```python
from build123d import *

# Parameters (mm, degrees)
F0_W     = 100
F0_H     = 100
F2_DEPTH = 15
F1_R     = 25
F3_DEPTH = 15.001
F4_R     = 8
F5_DEPTH = 15.001
F7_D     = 3.3
F7_DEPTH = 13.5
F7_TIP   = 0.9914200214


with BuildPart() as f2:
    # F0 (on Front) → F2 (new body)
    with BuildSketch(Plane.XZ):
        Rectangle(F0_W, F0_H)
    extrude(amount=F2_DEPTH)

    # F1 (on Front) → F3 (cut, through all)
    with BuildSketch(Plane.XZ):
        Circle(F1_R)
    extrude(amount=F3_DEPTH, mode=Mode.SUBTRACT)

    # F4 (on Front) → F5 (cut, through all)
    with BuildSketch(Plane.XZ):
        with Locations((0, 39.0632459029)):
            Circle(F4_R)
    extrude(amount=F5_DEPTH, mode=Mode.SUBTRACT)

    # F7
    with Locations(Plane.XY.offset(50)):
        with Locations((0, -8.1104654819)):
            Hole(F7_D / 2, depth=F7_DEPTH)
            with Locations((0, 0, -(F7_DEPTH + F7_TIP / 2))):  # 118° drill point
                Cone(0, F7_D / 2, F7_TIP, mode=Mode.SUBTRACT)


solid = f2.part
```
Design review of the part built by this model. Coordinates are the model's own, in mm. Coordinates: 2 decimals unless noted, no trailing zeros. Loops run counter-clockwise (first coordinate to the right, second up) from the corner with the lowest first, then second, coordinate; pieces in that order, holes last. Notation, with made-up numbers: (24.5, 79) -> (38.5, 79) arc R27 cw to (38.5, 96) -> close; hole circle Ø11 at (34.5, 83). An arc over 180 degrees is marked (long way). Answer as a JSON object with one key per item and string values.
Q1. Take a section at C-C on x = -4. Give the boundary of the cut face in (y, z).
Answer block:
{"outline": "(-15, -50) -> (0, -50) -> (0, -24.68) -> (-15, -24.68) -> close; (-15, 24.68) -> (0, 24.68) -> (0, 32.14) -> (-15, 32.14) -> close; (-15, 45.99) -> (0, 45.99) -> (0, 50) -> (-15, 50) -> close"}
Q2. The part is to be moulded in two halves that separate along X. For faces 1 (the flat face through (-50, -7, -1)), 2 (the cylindrical face through (23.846, -7.395, 7.509)), 3 (the cylindrical face through (-1.524, -8.742, 48.421)), 4 (the flat face through (-1, -6, 50)), say which applies: +X half, -X half, draft (parallel to the pull), parting line (faces both ways), or undercut.
Answer block:
{"face 1": "-X half", "face 2": "undercut", "face 3": "undercut", "face 4": "draft"}
Q3. To check wall thickness, follow L1, parallel to Y at x = 0, z = 48.05; L2, parallel to Z at x = 0, y = -12; L3, parallel to Z at x = -5, y = -2. State the ranges of each line that lie inside material, in increasing order.
Answer block:
{"L1": "y = -15 to -9.76, -6.46 to 0", "L2": "z = -50 to -25, 25 to 31.06, 47.06 to 50", "L3": "z = -50 to -24.49, 24.49 to 32.82, 45.31 to 50"}
Q4. Take a section at D-D on y = -3.75. Give the boundary of the cut face in (x, z).
Answer block:
{"outline": "(-50, -50) -> (50, -50) -> (50, 50) -> (-50, 50) -> close; hole circle Ø50 at (0, 0); hole circle Ø16 at (0, 39.06)"}
Q5. Take a section at B-B on z = 0. Give the boundary of the cut face in (x, y), plus the area to 3 significant figures.
Answer block:
{"outline": "(-50, -15) -> (-25, -15) -> (-25, 0) -> (-50, 0) -> close; (25, -15) -> (50, -15) -> (50, 0) -> (25, 0) -> close", "area": "750 mm^2"}
Q6. Take a section at A-A on x = -15. Give the boundary of the cut face in (y, z).
Answer block:
{"outline": "(-15, -50) -> (0, -50) -> (0, -20) -> (-15, -20) -> close; (-15, 20) -> (0, 20) -> (0, 50) -> (-15, 50) -> close"}
